For this review, take the finished solid that the model builds, in its own axes (mm). Face numbers are marked on the shaded views. A direction names the side the tool comes from. Coordinates: 2 decimals unless noted, no trailing zeros. Write each loop counter-clockwise with the first axis right and the second up, starting at its lowest first coordinate (ties: lowest second). Pieces come first, ordered by that corner, then holes.
```python
from build123d import *

# Parameters (mm, degrees)
F0_R     = 300
F0_R_2   = 296
F1_DEPTH = 900
F4_R     = 50.52
F5_DEPTH = 250


with BuildPart() as f1:
    # F0 (on Front) → F1 (new body)
    with BuildSketch(Plane.XZ):
        with Locations((-1.797136, 0)):
            Circle(F0_R)
        with Locations((-1.797136, 0)):
            Circle(F0_R_2, mode=Mode.SUBTRACT)
    extrude(amount=F1_DEPTH)

    # F2 (on Right) → F3 (revolve)
    with BuildSketch(Plane.YZ):
        Polygon((209.546715, 0), (0, 0), (0, -300), (209.546715, -50.52), align=None)
    revolve(axis=Axis((0, 104.773358, 0), (0, 1, 0)))

    # F4 (on face) → F5 (cut)
    with BuildSketch(Plane(origin=(0, 209.546715, 0), x_dir=(-1, 0, 0), z_dir=(0, 1, 0))):
        Circle(F4_R)
    extrude(amount=-F5_DEPTH, mode=Mode.SUBTRACT)


solid = f1.part
```
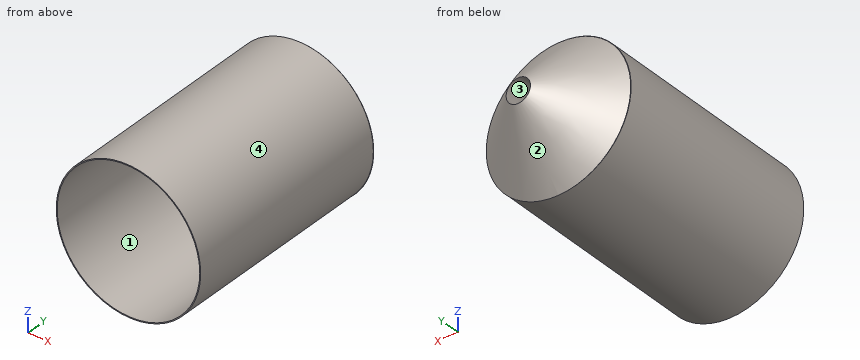
Q1. Add section A-A (z = 0). State the section outline as (x, y) points.
Ans:
outline: (-301.8, -900) - (-297.8, -900) - (-297.8, 0) - (-50.52, 0) - (-50.52, 209.55) - (-300, 0) - (-301.8, 0) - close; (50.52, 0) - (294.2, 0) - (294.2, -900) - (298.2, -900) - (298.2, 0) - (300, 0) - (50.52, 209.55) - close
Q2. Add section B-B (y = -228). State the section outline as (x, z) points.
Ans:
outline: circle Ø600 at (-1.8, 0); hole circle Ø592 at (-1.8, 0)
Q3. Tool access review of the marked faces 3 and 4: name each direction out of +Z, -Z, +X, -X, +Y, -Y from which nothing blocks a thin tool from reaching the whole face with its end or side.
Ans:
face 3: +Y, -Y
face 4: -Y
Q4. For probe 1 along Z at (x, y) = (0, 44); probe 2 along Z at (x, y) = (-147, -583); probe 3 along X at (y, z) = (-524.5, -60.5), list the stretches that pass through material, from the lowest coordinate up.
Ans:
probe 1: z = -247.61 to -50.52, 50.52 to 247.61
probe 2: z = -262.52 to -257.94, 257.94 to 262.52
probe 3: x = -295.63 to -291.55, 287.95 to 292.04
Q5. Draft analysis for pull direction Z (two halves, no side actions). For the marked faces 1 and 2, state which applies: +Z half, -Z half, draft (parallel to the pull), parting line (faces both ways), or undercut.
Ans:
face 1: undercut
face 2: parting line
Q6. Clearance check with flat-ended pins moving along their axes: pin 1 Ø8 at (y, z) = (-733.5, 189) entering from -X; pin 2 Ø1.5 at (x, y) = (-204.5, -74) entering from -Z; pin 3 Ø8 at (x, z) = (-117.5, -26) entering from +Y. State where each tip first meets the part, or that it passes through.
Ans:
pin 1: stops at x = -237.96
pin 2: stops at z = -221.84
pin 3: stops at y = 154.26
